from build123d import *

# Parameters (mm, degrees)
SKETCH1_W               = 38.1
SKETCH1_H               = 38.1
SKETCH1_W_2             = 31.75
SKETCH1_H_2             = 31.75
BOSS_EXTRUDE1_DEPTH     = 206.9
FILLET1_R               = 3.81
FILLET2_R               = 0.635
SKETCH2_R               = 3.175
CUT_EXTRUDE1_DEPTH      = 1
CUT_EXTRUDE1_DEPTH_BACK = 39.1
SKETCH3_R               = 3.175
CUT_EXTRUDE2_DEPTH      = 39.1


with BuildPart() as part:
    # Sketch1 → Boss-Extrude1 (new body, symmetric)
    with BuildSketch(Plane.XY):
        Rectangle(SKETCH1_W, SKETCH1_H)
        Rectangle(SKETCH1_W_2, SKETCH1_H_2, mode=Mode.SUBTRACT)
    extrude(amount=BOSS_EXTRUDE1_DEPTH, both=True)

    # Fillet1
    fillet1_edges = [part.edges().sort_by_distance(p)[0] for p in [
        (19.05, -19.05, 0),
        (-19.05, -19.05, 0),
        (-19.05, 19.05, 0),
        (19.05, 19.05, 0),
    ]]
    fillet(fillet1_edges, radius=FILLET1_R)

    # Fillet2
    fillet2_edges = [part.edges().sort_by_distance(p)[0] for p in [
        (15.875, 15.875, 0),
        (-15.875, 15.875, 0),
        (-15.875, -15.875, 0),
        (15.875, -15.875, 0),
    ]]
    fillet(fillet2_edges, radius=FILLET2_R)

    # Sketch2 → Cut-Extrude1 (cut, two sides)
    with BuildSketch(Plane(origin=(0, 19.05, 0), x_dir=(1, 0, 0), z_dir=(0, 1, 0))) as cut_extrude1_sk:
        with Locations((0, 202.85)):
            Circle(SKETCH2_R)
        with Locations((0, 134.75)):
            Circle(SKETCH2_R)
        with Locations((0, 53.0875)):
            Circle(SKETCH2_R)
        with Locations((0, -28.575)):
            Circle(SKETCH2_R)
        with Locations((0, -110.2375)):
            Circle(SKETCH2_R)
        with Locations((0, -191.9)):
            Circle(SKETCH2_R)
    extrude(amount=CUT_EXTRUDE1_DEPTH, mode=Mode.SUBTRACT)
    extrude(cut_extrude1_sk.sketch, amount=-CUT_EXTRUDE1_DEPTH_BACK, mode=Mode.SUBTRACT)

    # Sketch3 → Cut-Extrude2 (cut, through all)
    with BuildSketch(Plane(origin=(19.05, 0, 0), x_dir=(0, 0, -1), z_dir=(1, 0, 0))):
        with Locations((194.2, 10.05)):
            Circle(SKETCH3_R)
        with Locations((194.2, -10.05)):
            Circle(SKETCH3_R)
        with Locations((143.4, 10.05)):
            Circle(SKETCH3_R)
        with Locations((39.7, 10.05)):
            Circle(SKETCH3_R)
        with Locations((91.55, 10.05)):
            Circle(SKETCH3_R)
        with Locations((143.4, -10.05)):
            Circle(SKETCH3_R)
        with Locations((91.55, -10.05)):
            Circle(SKETCH3_R)
        with Locations((39.7, -10.05)):
            Circle(SKETCH3_R)
    extrude(amount=-CUT_EXTRUDE2_DEPTH, mode=Mode.SUBTRACT)


solid = part.part
Verification items for the finished model (mm, model axes). A direction names the side the tool comes from. Coordinates: 2 decimals unless noted, no trailing zeros. Order: outer loops, then holes, each group sorted by start corner. A loop starts at its lowest first (then second) coordinate and runs counter-clockwise, first axis right, second up.
1. Set-up check for faces 4 (the face through (-15.875, 0, 3)), 5 (the face through (0, 19.05, 3)): record each of +Z, -Z, +X, -X, +Y, -Y from which the full face is reachable in a straight line by a thin tool's end or side.
Results found:
face 4: +Z, -Z
face 5: +Z, -Z, +X, -X, +Y
2. Scan lines: line 1 (Y direction, x = 16, z = -194); line 2 (X direction, y = 4.5, z = 30) (3 decimals). Record each from-to range of solid material in increasing order.
Results found:
line 1: y = -18.97 to -13.22, -6.88 to 6.88, 13.22 to 18.97
line 2: x = -19.05 to -15.875, 15.875 to 19.05
3. Release check for a two-part mould opening along X. For faces 1 (the face through (19.05, 0, 3)), 2 (the face through (-0.69, -17.44, -199.75)), 3 (the face through (-17.44, 8.83, -146.33)) record: +X half, -X half, draft (parallel to the pull), parting line (faces both ways), or undercut.
Results found:
face 1: +X half
face 2: undercut
face 3: draft
4. Sectioned sample at A-A, the plane y = -3.5. Record the cut outline in (x, z) (3 decimals), and give its area (3 significant figures).
Results found:
outline: (-19.05, -206.9) - (-15.875, -206.9) - (-15.875, 206.9) - (-19.05, 206.9) - close; (15.875, -206.9) - (19.05, -206.9) - (19.05, 206.9) - (15.875, 206.9) - close
area: 2,630 mm2
5. Sectioned sample at C-C, the plane z = -164. Record the cut outline in (x, y) (3 decimals), and give its area (3 significant figures).
Results found:
outline: (-19.05, -15.24) arc R3.81 ccw to (-15.24, -19.05) - (15.24, -19.05) arc R3.81 ccw to (19.05, -15.24) - (19.05, 15.24) arc R3.81 ccw to (15.24, 19.05) - (-15.24, 19.05) arc R3.81 ccw to (-19.05, 15.24) - close; hole (-15.875, -15.24) arc R0.635 ccw to (-15.24, -15.875) - (15.24, -15.875) arc R0.635 ccw to (15.875, -15.24) - (15.875, 15.24) arc R0.635 ccw to (15.24, 15.875) - (-15.24, 15.875) arc R0.635 ccw to (-15.875, 15.24) - close
area: 431 mm2
6. Go/stop test with flat-tipped pins: pin 1 Ø8.5 at (x, z) = (0, -134.75) entering from -Y; pin 2 Ø5 at (x, z) = (0, -53.09) entering from +Y. Record where each tip stops, or that it passes through.
Results found:
pin 1: stops at y = -19.05
pin 2: passes through
